```python
from build123d import *

# Parameters (mm, degrees)
MAIN_BODY_SKETCH_W        = 45.5
MAIN_BODY_SKETCH_H        = 25
MAIN_BODY_EXTRUSION_DEPTH = 29
BOSS_EXTRUDE3_DEPTH       = 1
SKETCH8_W                 = 24
SKETCH8_H                 = 14
BOSS_EXTRUDE8_DEPTH       = 1
SKETCH3_R                 = 2.25
BOSS_EXTRUDE4_DEPTH       = 2
SKETCH6_R                 = 10
BOSS_EXTRUDE7_DEPTH       = 2.5
SKETCH7_R                 = 1.5
CUT_EXTRUDE1_DEPTH        = 2
SKETCH10_R                = 2.25
BOSS_EXTRUDE12_DEPTH      = 1
SKETCH11_R                = 10
BOSS_EXTRUDE13_DEPTH      = 2.1
SKETCH13_R                = 1.5
CUT_EXTRUDE3_DEPTH        = 2.1
BOSS_EXTRUDE9_DEPTH       = 2
SKETCH9_W                 = 5
SKETCH9_H                 = 20
CUT_EXTRUDE2_DEPTH        = 5
SKETCH4_R                 = 3
SKETCH4_R_2               = 1.25
BOSS_EXTRUDE10_DEPTH      = 4.1
SKETCH14_W                = 13.5
SKETCH14_H                = 17.856103011
BOSS_EXTRUDE14_DEPTH      = 2


with BuildPart() as part:
    # Main Body Sketch → Main Body Extrusion (new body)
    with BuildSketch(Plane(origin=(0, 0, 0), x_dir=(1, 0, 0), z_dir=(0, 1, 0))):
        Rectangle(MAIN_BODY_SKETCH_W, MAIN_BODY_SKETCH_H)
    extrude(amount=MAIN_BODY_EXTRUSION_DEPTH)

    # Sketch2 → Boss-Extrude3 (add)
    with BuildSketch(Plane(origin=(0, 29, 0), x_dir=(1, 0, 0), z_dir=(0, 1, 0))):
        with BuildLine():
            Line((-22.75, 12.5), (7.25, 12.5))
            Line((7.25, 12.5), (7.25, 10.099504938))
            ThreePointArc((7.25, 10.099504938), (1.25, 0), (7.25, -10.099504938))
            Line((7.25, -10.099504938), (7.25, -12.5))
            Line((7.25, -12.5), (-22.75, -12.5))
            Line((-22.75, -12.5), (-22.75, 12.5))
        make_face()
    extrude(amount=BOSS_EXTRUDE3_DEPTH)

    # Sketch8 → Boss-Extrude8 (add)
    with BuildSketch(Plane(origin=(0, 30, 0), x_dir=(1, 0, 0), z_dir=(0, 1, 0))):
        with Locations((-10.75, 0)):
            Rectangle(SKETCH8_W, SKETCH8_H)
    extrude(amount=BOSS_EXTRUDE8_DEPTH)

    # Sketch3 → Boss-Extrude4 (add)
    with BuildSketch(Plane(origin=(0, 29, 0), x_dir=(1, 0, 0), z_dir=(0, 1, 0))):
        with Locations(Location((12.75, 0, 0), (0, 0, 270))):
            Circle(SKETCH3_R)
    extrude(amount=BOSS_EXTRUDE4_DEPTH)

    # Sketch6 → Boss-Extrude7 (add)
    with BuildSketch(Plane(origin=(0, 31, 0), x_dir=(1, 0, 0), z_dir=(0, 1, 0))):
        with Locations(Location((12.75, 0, 0), (0, 0, 270))):
            Circle(SKETCH6_R)
    extrude(amount=BOSS_EXTRUDE7_DEPTH)

    # Sketch7 → Cut-Extrude1 (cut)
    with BuildSketch(Plane(origin=(0, 33.5, 0), x_dir=(1, 0, 0), z_dir=(0, 1, 0))):
        with Locations(Location((12.75, 7, 0), (0, 0, 270))):
            Circle(SKETCH7_R)
        with Locations(Location((12.75, -7, 0), (0, 0, 90))):
            Circle(SKETCH7_R)
        with Locations(Location((5.75, 0, 0), (0, 0, 270))):
            Circle(SKETCH7_R)
        with Locations(Location((19.75, 0, 0), (0, 0, 90))):
            Circle(SKETCH7_R)
    extrude(amount=-CUT_EXTRUDE1_DEPTH, mode=Mode.SUBTRACT)

    # Sketch10 → Boss-Extrude12 (add)
    with BuildSketch(Plane(origin=(0, 33.5, 0), x_dir=(1, 0, 0), z_dir=(0, 1, 0))):
        with Locations(Location((12.75, 0, 0), (0, 0, 270))):
            Circle(SKETCH10_R)
    extrude(amount=BOSS_EXTRUDE12_DEPTH)

    # Sketch11 → Boss-Extrude13 (add)
    with BuildSketch(Plane(origin=(0, 34.5, 0), x_dir=(1, 0, 0), z_dir=(0, 1, 0))):
        with Locations(Location((12.75, 0, 0), (0, 0, 270))):
            Circle(SKETCH11_R)
    extrude(amount=BOSS_EXTRUDE13_DEPTH)

    # Sketch13 → Cut-Extrude3 (cut)
    with BuildSketch(Plane(origin=(0, 36.6, 0), x_dir=(1, 0, 0), z_dir=(0, 1, 0))):
        with Locations(Location((12.75, 7, 0), (0, 0, 270))):
            Circle(SKETCH13_R)
        with Locations(Location((5.75, 0, 0), (0, 0, 270))):
            Circle(SKETCH13_R)
        with Locations(Location((12.75, -7, 0), (0, 0, 90))):
            Circle(SKETCH13_R)
        with Locations(Location((19.75, 0, 0), (0, 0, 90))):
            Circle(SKETCH13_R)
    extrude(amount=-CUT_EXTRUDE3_DEPTH, mode=Mode.SUBTRACT)

    # Sketch5 → Boss-Extrude9 (add)
    with BuildSketch(Plane.XZ):
        Polygon((-4, 12.5), (-22.75, 12.5), (-22.75, -12.5), (-4, -12.5), (-4, -10), (-4, 0), (-4, 10), align=None)
        Polygon((7, 12.5), (-4, 12.5), (-4, 10), (1, 10), (1, 6.5), (3.5, 6.5), (7, 10), align=None)
        Polygon((-4, -10), (-4, -12.5), (7, -12.5), (7, -10), (3.5, -6.5), (1, -6.5), (1, -10), align=None)
    extrude(amount=BOSS_EXTRUDE9_DEPTH)

    # Sketch9 → Cut-Extrude2 (cut)
    with BuildSketch(Plane.XZ):
        with Locations((-1.5, 0)):
            Rectangle(SKETCH9_W, SKETCH9_H)
    extrude(amount=-CUT_EXTRUDE2_DEPTH, mode=Mode.SUBTRACT)

    # Sketch4 → Boss-Extrude10 (add)
    with BuildSketch(Plane.XZ):
        with Locations(Location((12.5, 0, 0), (0, 0, 90))):
            Circle(SKETCH4_R)
        with Locations(Location((12.5, 0, 0), (0, 0, 270))):
            Circle(SKETCH4_R_2, mode=Mode.SUBTRACT)
    extrude(amount=BOSS_EXTRUDE10_DEPTH)

    # Sketch14 → Boss-Extrude14 (add)
    with BuildSketch(Plane.XZ.offset(2)):
        with Locations((-10.75, -0.020714737)):
            Rectangle(SKETCH14_W, SKETCH14_H)
    extrude(amount=BOSS_EXTRUDE14_DEPTH)


solid = part.part
```
Check sheet for the modelled part. Datum: model origin and axes. Units: mm. A direction names the side the tool comes from. Coordinates: 2 decimals unless noted, no trailing zeros. Order: outer loops, then holes, each group sorted by start corner. A loop starts at its lowest first (then second) coordinate and runs counter-clockwise, first axis right, second up. Notation, with made-up numbers: M 22.25,-5 L 73.25,-5 A33 ccw 73.25,29 Z; hole C -17,70.25 d5. An arc over 180 degrees is marked long. Write each question's results on one line, items separated by ' | '. Start each with the question number.
1. Access from +Z, -Z, +X, -X, +Y, -Y to the whole of each face (thin tool, end or side, straight path). Record for faces 1 (the face through (-10.9, 30.5, -7)), 2 (the face through (6, 31.5, 0)), 3 (the face through (5, -1, -8)), 4 (the face through (7, -1, 11)), 5 (the face through (12, 0, 0)).
2. Material ranges on probe 1 along Y at (x, z) = (8, 5.5); probe 2 along X at (y, z) = (2, 7.75); probe 3 along X at (y, z) = (33, 0.5), recorded low to high.
3. Cross-section at C-C on z = 3.75. Record the cut outline in (x, y), and give its area (3 significant figures).
4. Cross-section at D-D on x = -1. Record the cut outline in (y, z), and give its area (3 significant figures).
5. Go/stop test with flat-tipped pins: P1, Ø1.5, axis at x = -13.5, z = 2.5, coming from the +Y side; P2, Ø1, axis at y = -1, z = -11, coming from the +X side; P3, Ø2.5, axis at x = 5.75, z = 0, coming from the -Y side. Record where each tip stops, or that it passes through.
6. Cross-section at A-A on y = 2. Record the cut outline in (x, z).
7. Mould release check, pull along Z, two halves, no side actions. Record for faces 6 (the face through (-11, -3, -8.949)), 7 (the face through (-8, 30, 9)), 8 (the face through (14, 29, 3)): +Z half, -Z half, draft (parallel to the pull), parting line (faces both ways), or undercut.
8. Cross-section at B-B on x = 20.5. Record the cut outline in (y, z).
Checks:
1) face 1: -Z, +X, -X, +Y | face 2: +Y | face 3: +X, -Y | face 4: +Z, -Z, +X, -Y | face 5: -Y
2) probe 1: y = 0 to 29, 31 to 33.5, 34.5 to 36.6 | probe 2: x = -22.75 to -4, 1 to 22.75 | probe 3: x = 2.76 to 4.34, 7.16 to 18.34, 21.16 to 22.74
3) outline: M -22.75,-2 L -17.5,-2 L -17.5,-4 L -4,-4 L -4,5 L 1,5 L 1,0 L 22.75,0 L 22.75,29 L 1.88,29 L 1.88,30 L 1.25,30 L 1.25,31 L -22.75,31 Z; M 3.48,31 L 22.02,31 L 22.02,33.5 L 3.48,33.5 Z; M 3.48,34.5 L 22.02,34.5 L 22.02,36.6 L 3.48,36.6 Z | area: 1,490 mm²
4) outline: M -2,-12.5 L 30,-12.5 L 30,-7 L 31,-7 L 31,7 L 30,7 L 30,12.5 L -2,12.5 L -2,10 L 5,10 L 5,-10 L -2,-10 Z | area: 674 mm²
5) P1: stops at y = 31 | P2: stops at x = 7 | P3: stops at y = 0
6) outline: M -22.75,-12.5 L 22.75,-12.5 L 22.75,12.5 L -22.75,12.5 Z; hole M -4,-10 L 1,-10 L 1,10 L -4,10 Z
7) face 6: -Z half | face 7: draft | face 8: undercut
8) outline: M 0,-12.5 L 29,-12.5 L 29,12.5 L 0,12.5 Z; M 31,-6.32 L 33.5,-6.32 L 33.5,-1.3 L 31.5,-1.3 L 31.5,1.3 L 33.5,1.3 L 33.5,6.32 L 31,6.32 Z; M 34.5,-6.32 L 36.6,-6.32 L 36.6,-1.3 L 34.5,-1.3 Z; M 34.5,1.3 L 36.6,1.3 L 36.6,6.32 L 34.5,6.32 Z
